Source: CAD feature listing. Evaluate the final solid. Frame: model axes, mm. A direction names the side the tool comes from. Round coordinates to 2 decimals unless told otherwise and drop trailing zeros. Write each loop counter-clockwise with the first axis right and the second up, starting at its lowest first coordinate (ties: lowest second). Pieces come first, ordered by that corner, then holes.
Autodesk Inventor part; units mm, degrees
ref_plane "YZ Plane" through (0, 0, 0) normal (1, 0, 0) x (0, 1, 0)
ref_plane "XZ Plane" through (0, 0, 0) normal (0, 1, 0) x (-1, 0, 0)
ref_plane "XY Plane" through (0, 0, 0) normal (0, 0, 1) x (1, 0, 0)
sketch "Sketch2" plane through (0, 0, 0) normal (0, 0, 1) x (1, 0, 0)
  line L0 (0, 0) -> (76.2, 0)
  line L1 (76.2, 0) -> (76.2, 38.1)
  line L2 (0, 38.1) -> (0, 0)
  line L3 (76.2, 38.1) -> (0, 38.1)
  dimension "d0" = 76.2
  dimension "d1" = 38.1
extrude "Extrusion_channel" add sketch "Sketch2" along normal blind 177.8
sketch "Sketch3" plane through (76.2, 0, 0) normal (1, 0, 0) x (0, 0, -1)
  circle A0 centre (-12.7, 9.4234) radius 2.9464
  circle A1 centre (-12.7, 26.5334) radius 2.9464
  line L0 (0, 0) -> (-177.8, 0)
  line L1 (0, 0) -> (0, 38.1)
  circle A2 centre (-83.312, 9.4234) radius 2.9464
  circle A3 centre (-83.312, 26.5334) radius 2.9464
  line L2 (-78.486, 38.1) -> (-17.526, 38.1)
  line L3 (-17.526, 38.1) -> (-17.526, 3.175)
  line L4 (-17.526, 3.175) -> (-78.486, 3.175)
  line L5 (-78.486, 3.175) -> (-78.486, 38.1)
  line L6 (-78.486, 38.1) -> (-17.526, 3.175) construction
  line L7 (-17.526, 38.1) -> (-78.486, 3.175) construction
  line L8 (0, 38.1) -> (-177.8, 38.1)
  line L9 (-88.9, 38.1) -> (-88.9, 0)
  circle A4 centre (-165.1, 9.4234) radius 2.9464
  circle A5 centre (-165.1, 26.5334) radius 2.9464
  line L10 (-177.8, 0) -> (-177.8, 38.1)
  circle A6 centre (-94.488, 9.4234) radius 2.9464
  circle A7 centre (-94.488, 26.5334) radius 2.9464
  line L11 (-99.314, 38.1) -> (-160.274, 38.1)
  line L12 (-160.274, 38.1) -> (-160.274, 3.175)
  line L13 (-160.274, 3.175) -> (-99.314, 3.175)
  line L14 (-99.314, 3.175) -> (-99.314, 38.1)
  line L15 (-99.314, 38.1) -> (-160.274, 3.175) construction
  line L16 (-160.274, 38.1) -> (-99.314, 3.175) construction
  point P0 (-48.006, 20.6375)
  point P1 (-129.794, 20.6375)
  dimension "d9" = 5.8928
  dimension "d10" = 5.8928
  dimension "d11" = 9.4234
  dimension "d12" = 17.11
  dimension "d13" = 12.7
  dimension "d14" = 5.8928
  dimension "d15" = 5.8928
  dimension "d16" = 70.612
  dimension "d17" = 60.96
  dimension "d18" = 34.925
  dimension "d19" = 35.306
  dimension "d20" = 3.175
extrude "Extrusion_mount" cut sketch "Sketch3" against normal blind 3.175 contours A0 | A1 | L3 L4 L5 L2 | L14 L13 L12 L8 | A2 | A3 | A4 | A5 | A6 | A7
sketch "Sketch8" plane through (0, 0, 0) normal (-1, 0, 0) x (0, 0, 1)
  line L0 (0, 0) -> (177.8, 0)
  line L1 (88.9, 0) -> (169.037, 38.1)
  line L2 (78.486, 38.1) -> (177.8, 38.1)
  circle A0 centre (30.166, 17.9784) radius 6.35
  line L3 (0, 38.1) -> (0, 0)
  circle A1 centre (65.7664, -56.9012) radius 6.35
  point P0 (99.314, 38.1)
  point P1 (160.274, 38.1)
  dimension "d26" = 12.7
  dimension "d27" = 17.9784
  dimension "d28" = 30.166
extrude "Extrusion_hole" cut sketch "Sketch8" against normal blind 3.175
sketch "Sketch9" plane through (0, 0, 0) normal (0, 0, -1) x (-1, 0, 0)
  line L0 (-3.175, 3.175) -> (-73.025, 3.175)
  line L1 (-73.025, 3.175) -> (-73.025, 34.925)
  line L2 (-73.025, 34.925) -> (-3.175, 34.925)
  line L3 (-3.175, 34.925) -> (-3.175, 3.175)
  point P0 (0, 0)
  dimension "d32" = 3.175
  dimension "d33" = 3.175
  dimension "d34" = 69.85
  dimension "d35" = 31.75
extrude "Extrusion_tube" cut sketch "Sketch9" against normal up to next
equation "\"d0\" = o_width"
equation "\"d1\" = height"
equation "\"d7\" = length"
equation "\"d9\" = hole_dia"
equation "\"d10\" = hole_dia"
equation "\"d11\" = hole_height"
equation "\"d12\" = hole_spacing"
equation "\"d13\" = end_space"
equation "\"d14\" = hole_dia"
equation "\"d15\" = hole_dia"
equation "\"d16\" = mount_spacing"
equation "\"d17\" = servo_space"
equation "\"d18\" = height - thickness"
equation "\"d20\" = thickness"
equation "\"d21\" = thickness"
equation "\"d26\" = mount_dia"
equation "\"d27\" = 0.5 * hole_spacing + hole_height"
equation "\"d28\" = servo_axis + end_space"
equation "\"d29\" = thickness"
equation "\"d34\" = o_width - 2 * thickness"
equation "\"d35\" = height - 2 * thickness"
equation "\"length\" = 177.8"
equation "\"o_width\" = 76.2"
equation "\"thickness\" = 3.175"
equation "\"i_width\" = o_width - 2 * thickness"
equation "\"height\" = 0.5 * o_width"
equation "\"servo_space\" = 60.96"
equation "\"mount_spacing\" = 70.612"
equation "\"hole_dia\" = 5.8928"
equation "\"end_space\" = 12.7"
equation "\"hole_spacing\" = 17.11"
equation "\"servo_axis\" = 17.466"
equation "\"mount_dia\" = 12.7"
properties part number "upper_leg"
1) Section query D-D on z = 84. Return the cut outline in (x, y) (3 decimals), then the cut area to 3 significant figures.
Taken from the geometry:
outline: (0, 0) - (76.2, 0) - (76.2, 6.558) - (73.025, 6.558) - (73.025, 3.175) - (3.175, 3.175) - (3.175, 34.925) - (73.025, 34.925) - (73.025, 29.398) - (76.2, 29.398) - (76.2, 38.1) - (0, 38.1) - close; (73.025, 12.288) - (76.2, 12.288) - (76.2, 23.668) - (73.025, 23.668) - close
area: 649 mm2
2) Material intervals for line 1 (Y direction, x = 74, z = 165); line 2 (X direction, y = 32, z = 11) (3 decimals); line 3 (Y direction, x = 10, z = 51) (3 decimals), sorted ascending.
Taken from the geometry:
line 1: y = 0 to 6.48, 12.37 to 23.59, 29.48 to 38.1
line 2: x = 0 to 3.175, 73.025 to 76.2
line 3: y = 0 to 3.175, 34.925 to 38.1
3) Section query C-C on z = 60.5. Return the cut outline in (x, y) (3 decimals), then the cut area to 3 significant figures.
Taken from the geometry:
outline: (0, 0) - (76.2, 0) - (76.2, 3.175) - (3.175, 3.175) - (3.175, 34.925) - (73.025, 34.925) - (73.025, 38.1) - (0, 38.1) - close
area: 575 mm2
4) Pull-direction query (X, two-part tool) for faces 6 (the face through (74.635, 6.547, 13.339)), 7 (the face through (0, 19, 88)), 8 (the face through (39, 34.925, 88)); classes: released by +X, released by -X, zero draft, split by the parting line, or undercut.
Taken from the geometry:
face 6: zero draft
face 7: released by -X
face 8: undercut
5) Reachability of faces 1 (the face through (73.025, 37, 130)), 2 (the face through (73.025, 19, 9)), 3 (the face through (74.635, 26.663, 168.044)), 4 (the face through (1.57, 19.89, 36.22)), 5 (the face through (76.2, 15, 88)) from +Z, -Z, +X, -X, +Y, -Y: full face, straight path, thin tool, end or side. Return the list, or none.
Taken from the geometry:
face 1: +X, +Y
face 2: +Z, -Z
face 3: +X
face 4: +X, -X
face 5: +Z, -Z, +X, +Y, -Y
6) Section query A-A on z = 12.7. Return the cut outline in (x, y) (3 decimals), then the cut area to 3 significant figures.
Taken from the geometry:
outline: (0, 0) - (76.2, 0) - (76.2, 6.477) - (73.025, 6.477) - (73.025, 3.175) - (3.175, 3.175) - (3.175, 34.925) - (73.025, 34.925) - (73.025, 29.48) - (76.2, 29.48) - (76.2, 38.1) - (0, 38.1) - close; (73.025, 12.37) - (76.2, 12.37) - (76.2, 23.587) - (73.025, 23.587) - close
area: 648 mm2
7) Section query B-B on x = 38.5. Return the cut outline in (y, z) (3 decimals).
Taken from the geometry:
outline: (0, 0) - (3.175, 0) - (3.175, 177.8) - (0, 177.8) - close; (34.925, 0) - (38.1, 0) - (38.1, 177.8) - (34.925, 177.8) - close
8) Contact query for flat-ended pins moving along their axis: P1, Ø3.5, axis at y = 26.53, z = 94.49, coming from the +X side (3 decimals); P2, Ø3.5, axis at y = 36.5, z = 123.5, coming from the +X side (3 decimals). Output: stop coordinate, or through.
Taken from the geometry:
P1: stops at x = 3.175
P2: stops at x = 73.025
